CAD build for the part. Positions are in the model's coordinates, mm. A direction names the side the tool comes from. Give positions to 0.01 mm unless a question says otherwise; leave off trailing zeros. Order: outer loops, then holes, each group sorted by start corner. A loop starts at its lowest first (then second) coordinate and runs counter-clockwise, first axis right, second up.
Autodesk Inventor part; units mm, degrees
ref_plane "YZ Plane" through (0, 0, 0) normal (1, 0, 0) x (0, 1, 0)
ref_plane "XZ Plane" through (0, 0, 0) normal (0, 1, 0) x (-1, 0, 0)
ref_plane "XY Plane" through (0, 0, 0) normal (0, 0, 1) x (1, 0, 0)
sketch "Sketch1" plane through (0, 0, 0) normal (0, 1, 0) x (-1, 0, 0)
  line L0 (0, 0) -> (-300, 0)
  line L1 (-300, 0) -> (-300, -120)
  line L2 (-300, -120) -> (0, -120)
  line L3 (0, -120) -> (0, 0)
  line L4 (-96.25, -114) -> (-258.25, -114)
  line L5 (-258.25, -114) -> (-258.25, -6)
  line L6 (-258.25, -6) -> (-96.25, -6)
  line L7 (-96.25, -6) -> (-96.25, -114)
  circle A0 centre (-10, -17.5) radius 3
  circle A1 centre (-49.075, -14.1) radius 3
  circle A2 centre (-64.25, -14.1) radius 1.5
  circle A3 centre (-83, -14.1) radius 5.5
  circle A4 centre (-64.25, -14.1) radius 5.85 construction
  line L8 (-46.075, -17.1) -> (-52.075, -17.1) construction
  line L9 (-52.075, -17.1) -> (-52.075, -11.1) construction
  line L10 (-52.075, -11.1) -> (-46.075, -11.1) construction
  line L11 (-46.075, -11.1) -> (-46.075, -17.1) construction
  line L12 (-76.25, -20.1) -> (-89.75, -20.1) construction
  line L13 (-89.75, -20.1) -> (-89.75, -8.1) construction
  line L14 (-89.75, -8.1) -> (-76.25, -8.1) construction
  line L15 (-76.25, -8.1) -> (-76.25, -20.1) construction
  line L16 (-7.75, -83.75) -> (-86.25, -83.75)
  line L17 (-86.25, -83.75) -> (-86.25, -32.25)
  line L18 (-86.25, -32.25) -> (-7.75, -32.25)
  line L19 (-7.75, -32.25) -> (-7.75, -83.75)
  line L20 (-8, -83.5) -> (-86, -83.5) construction
  line L21 (-86, -83.5) -> (-86, -32.5) construction
  line L22 (-86, -32.5) -> (-8, -32.5) construction
  line L23 (-8, -32.5) -> (-8, -83.5) construction
  line L24 (-0.5, -93) -> (-93.5, -93) construction
  line L25 (-93.5, -93) -> (-93.5, -6) construction
  line L26 (-93.5, -6) -> (-0.5, -6) construction
  line L27 (-0.5, -6) -> (-0.5, -93) construction
  point P0 (-49.075, -17.1)
  point P1 (-52.075, -14.1)
  point P2 (-83, -20.1)
  point P3 (-89.75, -14.1)
  point P4 (-47, -83.5)
  point P5 (-47, -83.75)
  point P6 (-86, -58)
  point P7 (-86.25, -58)
  dimension "d0" = 300
  dimension "d1" = 6
  dimension "d4" = 3
  dimension "d5" = 11
  dimension "d6" = 6
  dimension "d7" = 18.75
  dimension "d8" = 15.175
  dimension "d9" = 11.7
  dimension "d10" = 6
  dimension "d11" = 13.5
  dimension "d12" = 12
  dimension "d15" = 162
  dimension "d16" = 108
  dimension "d18" = 6
  dimension "d19" = 6
  dimension "d20" = 78.5
  dimension "d21" = 51.5
  dimension "d22" = 78
  dimension "d23" = 51
  dimension "d24" = 18.4
  dimension "d25" = 7.5
  dimension "d27" = 87
  dimension "d28" = 9.5
  dimension "d29" = 10
  dimension "d30" = 0.5
  dimension "d33" = 6
  dimension "d34" = 15
  dimension "d35" = 9.5
  dimension "d36" = 10.5
  dimension "d37" = 93
extrude "Extrusion1" add sketch "Sketch1" along normal blind 6.5
sketch "Sketch2" plane through (0, 6.5, 0) normal (0, 1, 0) x (1, 0, 0)
  line L0 (7.75, 83.75) -> (86.25, 83.75)
  circle A0 centre (14.518, 104.846) radius 3
  circle A1 centre (32.775, 104.846) radius 3
  circle A2 centre (60.989, 104.846) radius 3
  circle A3 centre (78.996, 104.846) radius 3
  circle A4 centre (48.582, 104.846) radius 3
  circle A5 centre (80.796, 97.346) radius 1.5
  line L1 (9, 109.85) -> (85, 109.85) construction
  line L2 (85, 109.85) -> (85, 93.75) construction
  line L3 (85, 93.75) -> (9, 93.75) construction
  line L4 (9, 93.75) -> (9, 109.85) construction
  point P0 (47, 83.75)
  point P1 (47, 93.75)
  dimension "d38" = 6
  dimension "d39" = 18.257
  dimension "d40" = 15.807
  dimension "d41" = 12.407
  dimension "d42" = 18.007
  dimension "d43" = 3
  dimension "d44" = 1.8
  dimension "d45" = 7.5
  dimension "d46" = 76
  dimension "d47" = 16.1
  dimension "d48" = 5.004
  dimension "d49" = 5.518
  dimension "d50" = 10
extrude "Extrusion2" cut sketch "Sketch2" against normal through all
sketch "Sketch3" plane through (0, 6.5, 0) normal (0, 1, 0) x (1, 0, 0)
  line L0 (0, 0) -> (300, 0)
  line L1 (300, 120) -> (0, 120)
  line L2 (0, 120) -> (0, 0)
  line L3 (0, 96) -> (-4.5, 96)
  line L4 (-6.5, 94) -> (-6.5, 90)
  line L5 (-4.5, 88) -> (0, 88)
  line L6 (0, 88) -> (0, 96)
  line L7 (0, 64) -> (-4.5, 64)
  line L8 (-6.5, 62) -> (-6.5, 58)
  line L9 (-4.5, 56) -> (0, 56)
  line L10 (0, 56) -> (0, 64)
  line L11 (0, 32) -> (-4.5, 32)
  line L12 (-6.5, 30) -> (-6.5, 26)
  line L13 (-4.5, 24) -> (0, 24)
  line L14 (0, 24) -> (0, 32)
  line L15 (150, 120) -> (150, 0) construction
  arc A0 (-4.5, 96) -> (-6.5, 94) centre (-4.5, 94) ccw
  arc A1 (-6.5, 90) -> (-4.5, 88) centre (-4.5, 90) ccw
  arc A2 (-4.5, 64) -> (-6.5, 62) centre (-4.5, 62) ccw
  arc A3 (-6.5, 58) -> (-4.5, 56) centre (-4.5, 58) ccw
  arc A4 (-4.5, 32) -> (-6.5, 30) centre (-4.5, 30) ccw
  arc A5 (-6.5, 26) -> (-4.5, 24) centre (-4.5, 26) ccw
  line L16 (-2.25, 96) -> (-2.25, 120) construction
  line L17 (-2.25, 88) -> (-2.25, 64) construction
  line L18 (-2.25, 56) -> (-2.25, 32) construction
  line L19 (-2.25, 24) -> (-2.25, 0) construction
  line L20 (300, 96) -> (304.5, 96)
  line L21 (306.5, 94) -> (306.5, 90)
  line L22 (304.5, 88) -> (300, 88)
  line L23 (300, 88) -> (300, 96)
  line L24 (300, 64) -> (304.5, 64)
  line L25 (306.5, 62) -> (306.5, 58)
  line L26 (304.5, 56) -> (300, 56)
  line L27 (300, 56) -> (300, 64)
  line L28 (300, 32) -> (304.5, 32)
  line L29 (306.5, 30) -> (306.5, 26)
  line L30 (304.5, 24) -> (300, 24)
  line L31 (300, 24) -> (300, 32)
  arc A6 (306.5, 94) -> (304.5, 96) centre (304.5, 94) ccw
  arc A7 (304.5, 88) -> (306.5, 90) centre (304.5, 90) ccw
  arc A8 (306.5, 62) -> (304.5, 64) centre (304.5, 62) ccw
  arc A9 (304.5, 56) -> (306.5, 58) centre (304.5, 58) ccw
  arc A10 (306.5, 30) -> (304.5, 32) centre (304.5, 30) ccw
  arc A11 (304.5, 24) -> (306.5, 26) centre (304.5, 26) ccw
  point P0 (302.25, 96)
  point P1 (302.25, 88)
  point P2 (302.25, 64)
  point P3 (302.25, 56)
  point P4 (302.25, 32)
  point P5 (302.25, 24)
  dimension "d53" = 2
  dimension "d54" = 8
  dimension "d55" = 8
  dimension "d56" = 8
  dimension "d57" = 6.5
extrude "Extrusion3" add sketch "Sketch3" against normal blind 6.5
sketch "Sketch4" plane through (0, 6.5, 0) normal (0, 1, 0) x (1, 0, 0)
  circle A0 centre (80.796, 97.346) radius 1.5
extrude "Extrusion4" add sketch "Sketch4" against normal blind 6.5
properties part number "main_lcd_front_2" material "Plywood, Finish"
Item 1: Wall check: L1, parallel to Z at x = 64.25, y = 3.5; L2, parallel to X at y = 3.25, z = -58; L3, parallel to X at y = 6, z = -39. Give the ranges that are in metal, low to high.
Item 2: Two-plate mould, pull along X, no slides. Class faces 1 (the face through (148, 3, 0)), 2 (the face through (10.65, 3.2, -14.57)), 3 (the face through (300, 3, -44)): released by +X, released by -X, zero draft, split by the parting line, or undercut.
Item 3: Slice it at C-C (x = 219.5). Give the cut face in (y, z), and give its area (3 significant figures).
Item 4: Slice it at A-A (x = 70). Give the cut face in (y, z).
Item 5: Slice it at B-B (z = -76.5). Give the cut face in (x, y).
Item 6: Slice it at D-D (y = 3.25). State how many separate pieces and enclosed holes the cut face has, and give its area (3 significant figures).
Item 7: Tool access for faces 4 (the face through (178, 3, -6)), 5 (the face through (300, 3, -76)), 6 (the face through (300, 3, -12)), 7 (the face through (300, 3, -108)): list every direction of +Z, -Z, +X, -X, +Y, -Y with a clear straight run to the whole face (end or side of a thin tool).
Item 8: Drop flat-ended pins along their axis: pin 1 Ø3 at (y, z) = (4, -112.5) entering from +X; pin 2 Ø3.5 at (x, y) = (301.5, 4.5) entering from -Z; pin 3 Ø2 at (y, z) = (2.5, -102.5) entering from -X; pin 4 Ø2 at (x, y) = (-2, 1.5) entering from +Z. Give the stop position or say it passes through.
A:
1. L1: z = -120 to -83.75, -32.25 to -15.6, -12.6 to 0
1. L2: x = -6.5 to 7.75, 86.25 to 96.25, 258.25 to 306.5
1. L3: x = 0 to 7.75, 86.25 to 96.25, 258.25 to 300
2. face 1: zero draft
2. face 2: undercut
2. face 3: released by +X
3. outline: (0, -120) - (6.5, -120) - (6.5, -114) - (0, -114) - close; (0, -6) - (6.5, -6) - (6.5, 0) - (0, 0) - close
3. area: 78.0 mm2
4. outline: (0, -120) - (6.5, -120) - (6.5, -83.75) - (0, -83.75) - close; (0, -32.25) - (6.5, -32.25) - (6.5, 0) - (0, 0) - close
5. outline: (0, 0) - (7.75, 0) - (7.75, 6.5) - (0, 6.5) - close; (86.25, 0) - (96.25, 0) - (96.25, 6.5) - (86.25, 6.5) - close; (258.25, 0) - (300, 0) - (300, 6.5) - (258.25, 6.5) - close
6. separate pieces: 1
6. enclosed holes: 11
6. area: 14,500 mm2
7. face 4: +Y, -Y
7. face 5: +X, +Y, -Y
7. face 6: +Z, +X, +Y, -Y
7. face 7: -Z, +X, +Y, -Y
8. pin 1: stops at x = 300
8. pin 2: stops at z = -120
8. pin 3: stops at x = 0
8. pin 4: stops at z = -24
